Read the model definition and answer for the solid it produces. Units are mm, in the model's axes. A direction names the side the tool comes from. Coordinates: 2 decimals unless noted, no trailing zeros. Order: outer loops, then holes, each group sorted by start corner. A loop starts at its lowest first (then second) coordinate and runs counter-clockwise, first axis right, second up. Notation, with made-up numbers: (43.25, -0.5) -> (81.25, -0.5) arc R18 cw to (81.25, 8.5) -> close; hole circle Ø7 at (-11.5, -6.5). An arc over 180 degrees is marked (long way). Answer in a Markdown table with one row per item.
from build123d import *

# Parameters (mm, degrees)
F0_R     = 13.037168
F1_DEPTH = 1
F2_DEPTH = 11.7
F4_DEPTH = 25
F5_R     = 9.452617


with BuildPart() as f1:
    # F0 (on Front) → F1 (new body)
    with BuildSketch(Plane.XZ):
        with BuildLine():
            Line((-25, -0.5), (25, -0.5))
            Line((25, -0.5), (25, 0.5))
            ThreePointArc((25, 0.5), (22.513025, 13.448456), (21.397779, 26.586331))
            ThreePointArc((21.397779, 26.586331), (7.155404, 36.033672), (-7.086971, 26.586331))
            ThreePointArc((-7.086971, 26.586331), (-11.727618, 10.579535), (-25, 0.5))
            Line((-25, 0.5), (-25, -0.5))
        make_face()
        with Locations((7.113422, 21.42911)):
            Circle(F0_R, mode=Mode.SUBTRACT)
        with Locations((7.113422, 21.42911)):
            Circle(F0_R)
    extrude(amount=F1_DEPTH)

    # F0 (on Front) → F2 (join)
    with BuildSketch(Plane.XZ):
        with BuildLine():
            Line((-25, -0.5), (25, -0.5))
            Line((25, -0.5), (25, 0.5))
            ThreePointArc((25, 0.5), (22.513025, 13.448456), (21.397779, 26.586331))
            ThreePointArc((21.397779, 26.586331), (7.155404, 36.033672), (-7.086971, 26.586331))
            ThreePointArc((-7.086971, 26.586331), (-11.727618, 10.579535), (-25, 0.5))
            Line((-25, 0.5), (-25, -0.5))
        make_face()
        with Locations((7.113422, 21.42911)):
            Circle(F0_R, mode=Mode.SUBTRACT)
    extrude(amount=-F2_DEPTH)

    # F3 (on face) → F4 (cut)
    with BuildSketch(Plane(origin=(0, 11.7, 0), x_dir=(-1, 0, 0), z_dir=(0, 1, 0))):
        with BuildLine():
            Line((-17.169921, 6.49079), (-21.374672, 7.891529))
            ThreePointArc((-21.374672, 7.891529), (-21.997455, 4.687271), (-22.702033, 1.5))
            Line((-22.702033, 1.5), (-18.964415, 1.5))
            Line((-18.964415, 1.5), (-17.169921, 6.49079))
        make_face()
        with BuildLine():
            Line((-16.703859, 7.786989), (-16.126572, 9.392519))
            ThreePointArc((-16.126572, 9.392519), (-18.523006, 11.634326), (-20.376068, 14.342601))
            ThreePointArc((-20.376068, 14.342601), (-20.721893, 11.849812), (-21.116834, 9.364331))
            Line((-21.116834, 9.364331), (-16.703859, 7.786989))
        make_face()
        with BuildLine():
            Line((5.783263, 6.227552), (3.645503, 10.923782))
            ThreePointArc((3.645503, 10.923782), (-5.436746, 6.485712), (-15.276698, 8.800677))
            Line((-15.276698, 8.800677), (-15.762202, 7.450409))
            Line((-15.762202, 7.450409), (-2.188527, 2.598733))
            Line((-2.188527, 2.598733), (5.783263, 6.227552))
        make_face()
        Polygon((-17.901738, 1.5), (-2.994426, 1.5), (-2.994426, 1.768471), (-16.220917, 6.174646), align=None)
        Polygon((-1.334743, 1.5), (7.935281, 1.5), (6.197565, 5.317413), (-1.334743, 1.888649), align=None)
        with BuildLine():
            ThreePointArc((18.324978, 1.5), (14.605987, 4.307356), (11.393648, 7.682709))
            Line((11.393648, 7.682709), (7.107705, 5.731715))
            Line((7.107705, 5.731715), (9.034014, 1.5))
            Line((9.034014, 1.5), (18.324978, 1.5))
        make_face()
        with BuildLine():
            ThreePointArc((10.762688, 8.494224), (8.524386, 11.985495), (6.815958, 15.764417))
            ThreePointArc((6.815958, 15.764417), (5.755764, 13.650907), (4.377367, 11.729721))
            Line((4.377367, 11.729721), (6.693402, 6.641855))
            Line((6.693402, 6.641855), (10.762688, 8.494224))
        make_face()
    extrude(amount=-F4_DEPTH, mode=Mode.SUBTRACT)

    # F5
    f5_edges = [f1.edges().sort_by_distance(p)[0] for p in [
        (-7.086971, 5.35, 26.586331),
        (21.397779, 5.35, 26.586331),
    ]]
    fillet(f5_edges, radius=F5_R)


solid = f1.part
Q1. The part is cut by section C-C (x = -1). Write down the section's boundary in (y, z).
Outcome:
| item | result |
|---|---|
| outline | (-1, -0.5) -> (11.7, -0.5) -> (11.7, 1.5) -> (-1, 1.5) -> close; (-1, 2.95) -> (11.7, 2.95) -> (11.7, 4.05) -> (-1, 4.05) -> close; (-1, 8.77) -> (11.7, 8.77) -> (11.7, 11.22) -> (0, 11.22) -> (0, 31.63) -> (11.7, 31.63) -> (11.7, 33.71) -> (-1, 33.71) -> close |
Q2. For a pull along X with two mould halves and no side action, classify faces 1 (the face through (7.54, 5.26, 36.03)), 2 (the face through (5, -1, 18)), 3 (the face through (17.05, 5.44, 3.87)), 4 (the face through (-9.28, 5.44, 6.72)) as pulls with the +X half, pulls with the -X half, needs draft (parallel to the pull), parting line crosses it, or undercut.
Outcome:
| item | result |
|---|---|
| face 1 | parting line crosses it |
| face 2 | needs draft |
| face 3 | undercut |
| face 4 | undercut |
Q3. The part is cut by section D-D (z = 22). Write down the section's boundary in (x, y).
Outcome:
| item | result |
|---|---|
| outline | (-7.31, -1) -> (21.63, -1) -> (21.63, 11.7) -> (20.14, 11.7) -> (20.14, 0) -> (-5.91, 0) -> (-5.91, 11.7) -> (-7.31, 11.7) -> close |
Q4. Consider line 1 (Z direction, x = -3, y = 10); line 2 (Z direction, x = 8, y = 4.25); line 3 (Z direction, x = 2, y = 11). Determine where each line is inside the solid, lowest interval first.
Outcome:
| item | result |
|---|---|
| line 1 | -0.5 to 1.5, 3.86 to 4.96, 10.3 to 13.2, 29.66 to 32.23 |
| line 2 | -0.5 to 1.5, 3.44 to 4.68, 6.42 to 8.42, 34.44 to 36.01 |
| line 3 | -0.5 to 2.68, 7.29 to 9.44, 33.42 to 35.15 |
Q5. The part is cut by section A-A (x = -16.5). Write down the section's boundary in (y, z).
Outcome:
| item | result |
|---|---|
| outline | (-1, -0.5) -> (11.7, -0.5) -> (11.7, 1.5) -> (-1, 1.5) -> close; (-1, 2.76) -> (11.7, 2.76) -> (11.7, 5.31) -> (-1, 5.31) -> close |
Q6. Given pin 1 (1.1 mm diameter, centred on x = 21, y = 4.5, fed in from +Z); pin 2 (1.5 mm diameter, centred on x = -1, z = 12.5, fed in from +Y); pin 3 (3 mm diameter, centred on x = -4, y = 3.5, fed in from +Z), each flat-ended and moving along its own axis, determine where each tip first touches the part or whether it passes through.
Outcome:
| item | result |
|---|---|
| pin 1 | z = 28.39 |
| pin 2 | y = 0 |
| pin 3 | z = 32.65 |
Q7. For faces 5 (the face through (-25, 5, 0)), 6 (the face through (-5.91, 5.77, 22)), 7 (the face through (11, 5, 1.5)), determine the directions among +Z, -Z, +X, -X, +Y, -Y from which every point of the face is accessible in a straight line to the end or side of a thin tool.
Outcome:
| item | result |
|---|---|
| face 5 | +Z, -Z, -X, +Y, -Y |
| face 6 | +Y |
| face 7 | +Y, -Y |
Q8. The part is cut by section B-B (z = 15). Write down the section's boundary in (x, y).
Outcome:
| item | result |
|---|---|
| outline | (-9.28, -1) -> (-7.11, -1) -> (-7.11, 11.7) -> (-9.28, 11.7) -> close; (-6.48, -1) -> (22.31, -1) -> (22.31, 11.7) -> (18.46, 11.7) -> (18.46, 0) -> (-4.23, 0) -> (-4.23, 11.7) -> (-6.48, 11.7) -> close |
